```python
from build123d import *

# Parameters (mm, degrees)
BASEHEAD_DEPTH          = 18
SKETCH4_W               = 0.8
SKETCH4_H               = 11.547005384
CUT_EXTRUDE1_DEPTH      = 90.315918702
CUT_EXTRUDE1_DEPTH_BACK = 90.315918702
SKETCH6_R               = 15


# Read off the part's stored shape, not the designer's step: HeadChamfer
with BuildPart() as part:
    # Sketch1 → BaseHead (new body)
    with BuildSketch(Plane(origin=(0, 0, 0), x_dir=(0, 0, -1), z_dir=(1, 0, 0))):
        Polygon((10, 5.773502692), (10, -5.773502692), (0, -11.547005384), (-10, -5.773502692), (-10, 5.773502692), (0, 11.547005384), align=None)
    extrude(amount=BASEHEAD_DEPTH)

    # HeadChamfer outline → HeadChamfer (revolve, cut)
    with BuildSketch(Plane.YX):
        Polygon((11.547005388, 0.893163977), (10, 0), (11.547005388, 0), align=None)
    revolve(axis=Axis((0, 0, 0), (1, 0, 0)), mode=Mode.SUBTRACT)

    # HeadChamfer 2 outline → HeadChamfer 2 (revolve)
    with BuildSketch(Plane.YX):
        Polygon((6, 18), (6, 87), (5, 88), (0, 88), (0, 18), align=None)
    revolve(axis=Axis((0, 0, 0), (1, 0, 0)))

    # Sketch4 → BearingFace (revolve, cut)
    with BuildSketch(Plane.XY, mode=Mode.PRIVATE) as bearingface_sk:
        with Locations((17.6, 15.773502692)):
            Rectangle(SKETCH4_W, SKETCH4_H)
    revolve(bearingface_sk.sketch.rotate(Axis((0, 0, 0), (1, 0, 0)), 90), axis=Axis((0, 0, 0), (1, 0, 0)), mode=Mode.SUBTRACT)

    # Sketch6 → Cut-Extrude1 (cut, two sides: drawn at the far end of the back side and taken through both)
    with BuildSketch(Plane(origin=(0, 0, 0), x_dir=(1, 0, 0), z_dir=(0, 1, 0)).offset(-CUT_EXTRUDE1_DEPTH_BACK)):
        with Locations((50, 15)):
            Circle(SKETCH6_R)
    extrude(amount=CUT_EXTRUDE1_DEPTH + CUT_EXTRUDE1_DEPTH_BACK, mode=Mode.SUBTRACT)


solid = part.part
```
Verification items for the finished model (mm, model axes). A direction names the side the tool comes from. Give positions to 0.01 mm unless a question says otherwise; leave off trailing zeros. Write each loop counter-clockwise with the first axis right and the second up, starting at its lowest first coordinate (ties: lowest second). Pieces come first, ordered by that corner, then holes. Notation, with made-up numbers: (61.25, 55) - (81.25, 55) arc R24 cw to (81.25, 79) - close; hole circle Ø1 at (40, -29.5). An arc over 180 degrees is marked (long way). Put each result on its own line as item: value.
Q1. Section check A-A on x = 7.5. Record the cut outline in (y, z).
Result:
outline: (-11.55, 0) - (-5.77, -10) - (5.77, -10) - (11.55, 0) - (5.77, 10) - (-5.77, 10) - close
Q2. Section check B-B on x = 77. Record the cut outline in (y, z).
Result:
outline: circle Ø12 at (0, 0)
Q3. Depth check by flat-ended pin: P1, Ø8, axis at y = 6, z = 7, coming from the -X side; P2, Ø4, axis at y = -5.5, z = 8, coming from the +X side; P3, Ø2, axis at x = 56, z = 1, coming from the +Y side; P4, Ø8, axis at x = 56, z = 5, coming from the -Y side. Enter the tip coordinate at first touch or a pass-through.
Result:
P1: x = 0
P2: x = 18
P3: y = 6
P4: y = -5.92
Q4. Scan lines: probe 1 along X at (y, z) = (-6.5, -6.75); probe 2 along X at (y, z) = (-0.5, -4.25); probe 3 along Y at (x, z) = (12.5, -5). Record each from-to range of solid material in increasing order. Write a range as from..to.
Result:
probe 1: 0..18
probe 2: 0..39.54, 60.46..88
probe 3: -8.66..8.66
Q5. Section check D-D on x = 58.5. Record the cut outline in (y, z), and give its area (3 significant figures).
Result:
outline: (-5.39, -2.64) - (5.39, -2.64) arc R6 ccw (long way) to start
area: 87.2 mm2
Q6. Set-up check for faces 1 (the face through (17.2, -5, -9)), 2 (the face through (17.2, -5, 9)), 3 (the face through (17.2, 5, -9)), 4 (the face through (17.61, -0.44, -9.99)): record each of +Z, -Z, +X, -X, +Y, -Y from which the full face is reachable in a straight line by a thin tool's end or side.
Result:
face 1: -Z, +X, -Y
face 2: +Z, +X, -Y
face 3: -Z, +X, +Y
face 4: +X
